Work out the finished part from the listing and answer in its coordinate system (mm). Face numbers are marked on the shaded views. A direction names the side the tool comes from. Give positions to 0.01 mm unless a question says otherwise; leave off trailing zeros. Write each loop counter-clockwise with the first axis right and the second up, starting at its lowest first coordinate (ties: lowest second). Pieces come first, ordered by that corner, then holes. Notation, with made-up numbers: (43.25, 39) -> (83.25, 39) arc R22 cw to (83.25, 53) -> close; hole circle Ø5 at (3.5, 83). An arc over 180 degrees is marked (long way). Use a Markdown table: item, result. Add a question column.
Q1. Consider line 1 (X direction, y = 46.5, z = -4.75); line 2 (Z direction, x = -20, y = 37.25); line 3 (Y direction, x = -11.5, z = -6.25). Determine where each line is inside the solid, lowest interval first.
Q2. For a pull along X with two mould halves and no side action, classify the marked faces 5, 6 and 7 as pulls with the +X half, pulls with the -X half, needs draft (parallel to the pull), parting line crosses it, or undercut.
Q3. Section B-B, the plane y = 33.5 is taken. Give the vertices of the cut face in (x, z).
Q4. Each of these flat-tipped pins is pushed along its axis until it touches: pin 1 Ø1 at (x, z) = (18, 8.5) entering from -Y; pin 2 Ø4 at (y, z) = (35.5, -1.5) entering from +X; pin 3 Ø2.5 at (x, z) = (27.5, 5) entering from -Y. Where does it stop, or does it pass through?
Q5. Section C-C, the plane z = 10.25 is taken. Give the vertices of the cut face in (x, y).
Q6. Section D-D, the plane y = 23.5 is taken. Give the vertices of the cut face in (x, z).
Q7. Section A-A, the plane x = -14 is taken. Give the vertices of the cut face in (y, z), plus the area to 3 significant figures.
Q8. For the marked faces 1, 2, 3 and 4, determine the directions among +Z, -Z, +X, -X, +Y, -Y from which every point of the face is accessible in a straight line to the end or side of a thin tool.
from build123d import *

# Parameters (mm, degrees)
BOSS_EXTRUDE1_DEPTH                  = 12
F_2_7_2_7_DIAMETER_HOLE1_D           = 2.7
F_2_7_2_7_DIAMETER_HOLE1_DEPTH       = 8
F_2_7_2_7_DIAMETER_HOLE1_CSINK_D     = 2.75
F_2_7_2_7_DIAMETER_HOLE1_CSINK_ANGLE = 90
F_2_7_2_7_DIAMETER_HOLE1_TIP         = 0.811161836
F_2_7_2_7_DIAMETER_HOLE2_D           = 2.7
F_2_7_2_7_DIAMETER_HOLE2_DEPTH       = 8
F_2_7_2_7_DIAMETER_HOLE2_CSINK_D     = 2.75
F_2_7_2_7_DIAMETER_HOLE2_CSINK_ANGLE = 90
F_2_7_2_7_DIAMETER_HOLE2_TIP         = 0.811161836


with BuildPart() as part:
    # Sketch1 → Boss-Extrude1 (new, symmetric)
    with BuildSketch(Plane.XY):
        Polygon((0, 0), (-23, 0), (-31, 0), (-31, 77), (-23.404895261, 77), (32.5, 77), (32.5, 42), (24.5, 42), (24.5, 69), (-23, 69), (-23, 39.5), (-16, 39.5), (-16, 31.5), (0, 31.5), align=None)
    extrude(amount=BOSS_EXTRUDE1_DEPTH, both=True)

    # Ø2.7 (2.7) Diameter Hole1
    with Locations(Plane(origin=(0, 39.5, 0), x_dir=(1, 0, 0), z_dir=(0, 1, 0))):
        with Locations((-20, 4.75), (-20, -4.75)):
            CounterSinkHole(F_2_7_2_7_DIAMETER_HOLE1_D / 2, F_2_7_2_7_DIAMETER_HOLE1_CSINK_D / 2, depth=F_2_7_2_7_DIAMETER_HOLE1_DEPTH, counter_sink_angle=F_2_7_2_7_DIAMETER_HOLE1_CSINK_ANGLE)
            with Locations((0, 0, -(F_2_7_2_7_DIAMETER_HOLE1_DEPTH + F_2_7_2_7_DIAMETER_HOLE1_TIP / 2))):  # 118° drill point
                Cone(0, F_2_7_2_7_DIAMETER_HOLE1_D / 2, F_2_7_2_7_DIAMETER_HOLE1_TIP, mode=Mode.SUBTRACT)

    # Ø2.7 (2.7) Diameter Hole2
    with Locations(Plane(origin=(0, 42, 0), x_dir=(-1, 0, 0), z_dir=(0, -1, 0))):
        with Locations((-28.5, 4.75), (-28.5, -4.75)):
            CounterSinkHole(F_2_7_2_7_DIAMETER_HOLE2_D / 2, F_2_7_2_7_DIAMETER_HOLE2_CSINK_D / 2, depth=F_2_7_2_7_DIAMETER_HOLE2_DEPTH, counter_sink_angle=F_2_7_2_7_DIAMETER_HOLE2_CSINK_ANGLE)
            with Locations((0, 0, -(F_2_7_2_7_DIAMETER_HOLE2_DEPTH + F_2_7_2_7_DIAMETER_HOLE2_TIP / 2))):  # 118° drill point
                Cone(0, F_2_7_2_7_DIAMETER_HOLE2_D / 2, F_2_7_2_7_DIAMETER_HOLE2_TIP, mode=Mode.SUBTRACT)


solid = part.part
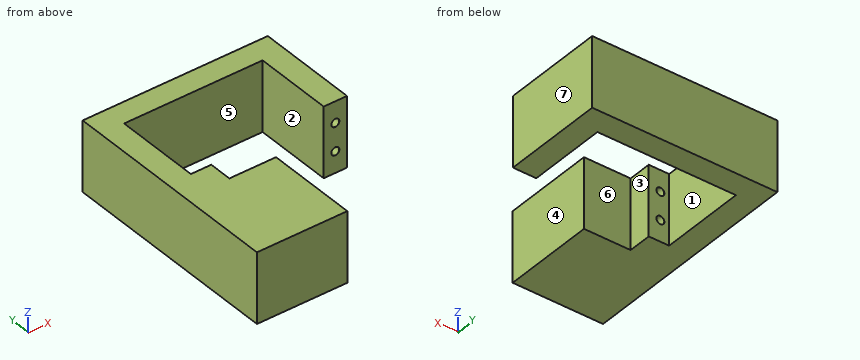
Result set:
| question | item | result |
|---|---|---|
| 1 | line 1 | x = -31 to -23, 24.5 to 27.15, 29.85 to 32.5 |
| 1 | line 2 | z = -12 to -6.1, -3.4 to 3.4, 6.1 to 12 |
| 1 | line 3 | y = 0 to 31.5, 69 to 77 |
| 2 | face 5 | undercut |
| 2 | face 6 | needs draft |
| 2 | face 7 | pulls with the +X half |
| 3 | outline | (-31, -12) -> (-16, -12) -> (-16, 12) -> (-31, 12) -> close; hole circle Ø2.7 at (-20, -4.75); hole circle Ø2.7 at (-20, 4.75) |
| 4 | pin 1 | stops at y = 69 |
| 4 | pin 2 | stops at x = -16 |
| 4 | pin 3 | stops at y = 42 |
| 5 | outline | (-31, 0) -> (0, 0) -> (0, 31.5) -> (-16, 31.5) -> (-16, 39.5) -> (-23, 39.5) -> (-23, 69) -> (24.5, 69) -> (24.5, 42) -> (32.5, 42) -> (32.5, 77) -> (-31, 77) -> close |
| 6 | outline | (-31, -12) -> (0, -12) -> (0, 12) -> (-31, 12) -> close |
| 7 | outline | (0, -12) -> (31.5, -12) -> (31.5, 12) -> (0, 12) -> close; (69, -12) -> (77, -12) -> (77, 12) -> (69, 12) -> close |
| 7 | area | 948 mm2 |
| 8 | face 1 | +Z, -Z |
| 8 | face 2 | +Z, -Z, -Y |
| 8 | face 3 | +Z, -Z, +X |
| 8 | face 4 | +Z, -Z, +X, -Y |
